Part model, mm, in its own coordinate system. Face numbers are marked on the shaded views. A direction names the side the tool comes from. Coordinates: 2 decimals unless noted, no trailing zeros. Loops run counter-clockwise (first coordinate to the right, second up) from the corner with the lowest first, then second, coordinate; pieces in that order, holes last. Notation, with made-up numbers: (18.5, -27) - (46.5, -27) arc R19 cw to (46.5, -11) - close; hole circle Ø10 at (42.25, -10.75). An arc over 180 degrees is marked (long way). Answer as CSV lines item,"result".
from build123d import *

# Parameters (mm, degrees)
F2_R     = 15
F3_DEPTH = 50.001
F5_DEPTH = 30
F7_DEPTH = 10
F8_R     = 5


with BuildPart() as f1:
    # F0 (on Top) → F1 (revolve)
    with BuildSketch(Plane.XY):
        Polygon((40, 0), (0, 0), (0, -15), (50, -15), (50, -6), (40, -6), align=None)
        Polygon((50, -15), (0, -15), (0, -30), (30, -30), (30, -50), (50, -50), align=None)
    revolve(axis=Axis((20, 0, 0), (-1, 0, 0)))

    # F2 (on face) → F3 (cut, through all)
    with BuildSketch(Plane(origin=(0, 0, 0), x_dir=(0, -1, 0), z_dir=(-1, 0, 0))):
        Circle(F2_R)
    extrude(amount=-F3_DEPTH, mode=Mode.SUBTRACT)

    # F4 (on face) → F5 (cut, through all)
    with BuildSketch(Plane(origin=(0, 0, 0), x_dir=(0, -1, 0), z_dir=(-1, 0, 0))):
        with BuildLine():
            Line((14.6969384567, -3), (18, -3))
            Line((18, -3), (18, 3))
            Line((18, 3), (14.6969384567, 3))
            ThreePointArc((14.6969384567, 3), (14.9240422951, 1.5076344301), (15, 0))
            ThreePointArc((15, 0), (14.9240422951, -1.5076344301), (14.6969384567, -3))
        make_face()
    extrude(amount=-F5_DEPTH, mode=Mode.SUBTRACT)

    # F6 (on face) → F7 (cut)
    with BuildSketch(Plane.YZ.offset(50)):
        with BuildLine():
            ThreePointArc((-49.638694584, 6), (-50, 0), (-49.638694584, -6))
            Line((-49.638694584, -6), (-13.7477270849, -6))
            ThreePointArc((-13.7477270849, -6), (-15, 0), (-13.7477270849, 6))
            Line((-13.7477270849, 6), (-49.638694584, 6))
        make_face()
        with BuildLine():
            Line((13.7477270849, -6), (49.638694584, -6))
            ThreePointArc((49.638694584, -6), (49.9095919098, -3.0054343115), (50, 0))
            ThreePointArc((50, 0), (49.9095919098, 3.0054343115), (49.638694584, 6))
            Line((49.638694584, 6), (13.7477270849, 6))
            ThreePointArc((13.7477270849, 6), (14.683594694, 3.0646446553), (15, 0))
            ThreePointArc((15, 0), (14.683594694, -3.0646446553), (13.7477270849, -6))
        make_face()
    extrude(amount=-F7_DEPTH, mode=Mode.SUBTRACT)

    # F8
    f8_edges = [f1.edges().sort_by_distance(p)[0] for p in [
        (30, 30, 0),
    ]]
    fillet(f8_edges, radius=F8_R)


solid = f1.part
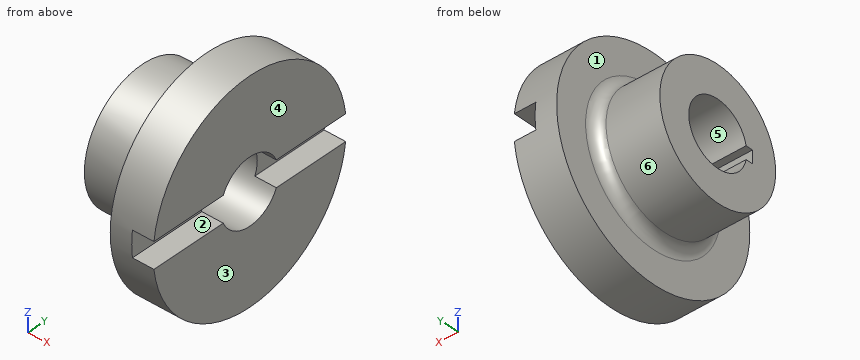
Q1. Saw through at A-A (y = 0). Give the cut face in (x, z).
Results:
outline,"(0, -30) - (25, -30) arc R5 cw to (30, -35) - (30, -50) - (50, -50) - (50, -15) - (0, -15) - close; (0, 15) - (50, 15) - (50, 50) - (30, 50) - (30, 35) arc R5 cw to (25, 30) - (0, 30) - close"
Q2. Flat gauge pins, fed straight in: pin 1 (2 mm diameter, centred on x = 40, y = 26.5, fed in from -Z); pin 2 (1.7 mm diameter, centred on y = -16, z = 1, fed in from -X); pin 3 (6 mm diameter, centred on x = 40.5, z = -8, fed in from +Y); pin 4 (24 mm diameter, centred on y = 0, z = 0, fed in from -X). Where does each tip first touch, or does it go through?
Results:
pin 1,"stops at z = -43.01"
pin 2,"stops at x = 30"
pin 3,"stops at y = 49.75"
pin 4,"passes through"
Q3. Saw through at C-C (x = 19). Give the cut face in (y, z).
Results:
outline,"circle Ø60 at (0, 0); hole (-18, -3) - (-14.7, -3) arc R15 ccw (long way) to (-14.7, 3) - (-18, 3) - close"
Q4. Saw through at B-B (z = 0). Give the cut face in (x, y).
Results:
outline,"(0, -30) - (25, -30) arc R5 cw to (30, -35) - (30, -50) - (40, -50) - (40, -15) - (30, -15) - (30, -18) - (0, -18) - close; (0, 15) - (40, 15) - (40, 50) - (30, 50) - (30, 35) arc R5 cw to (25, 30) - (0, 30) - close"
Q5. Two-plate mould, pull along Y, no slides. Class the marked faces 4, 5 and 6: released by +Y, released by -Y, zero draft, split by the parting line, or undercut.
Results:
face 4,"zero draft"
face 5,"undercut"
face 6,"split by the parting line"
Q6. Saw through at D-D (y = 40). Give the cut face in (x, z), then the cut area to 3 significant figures.
Results:
outline,"(30, -30) - (50, -30) - (50, -6) - (40, -6) - (40, 6) - (50, 6) - (50, 30) - (30, 30) - close"
area,"1,080 mm^2"
Q7. Which spindle directions (+Z, -Z, +X, -X, +Y, -Y) get a long thin tool onto all of the face, cutting with end or side? Do the marked faces 1, 2 and 3. Say none if no direction does.
Results:
face 1,"-X"
face 2,"+X, +Y, -Y"
face 3,"+Z, -Z, +X, +Y, -Y"
Q8. Wall check: L1, parallel to Z at x = 23, y = 0; L2, parallel to Z at x = 30.5, y = 0. Give the ranges that are in metal, low to high.
Results:
L1,"z = -30 to -15, 15 to 30"
L2,"z = -50 to -15, 15 to 50"
